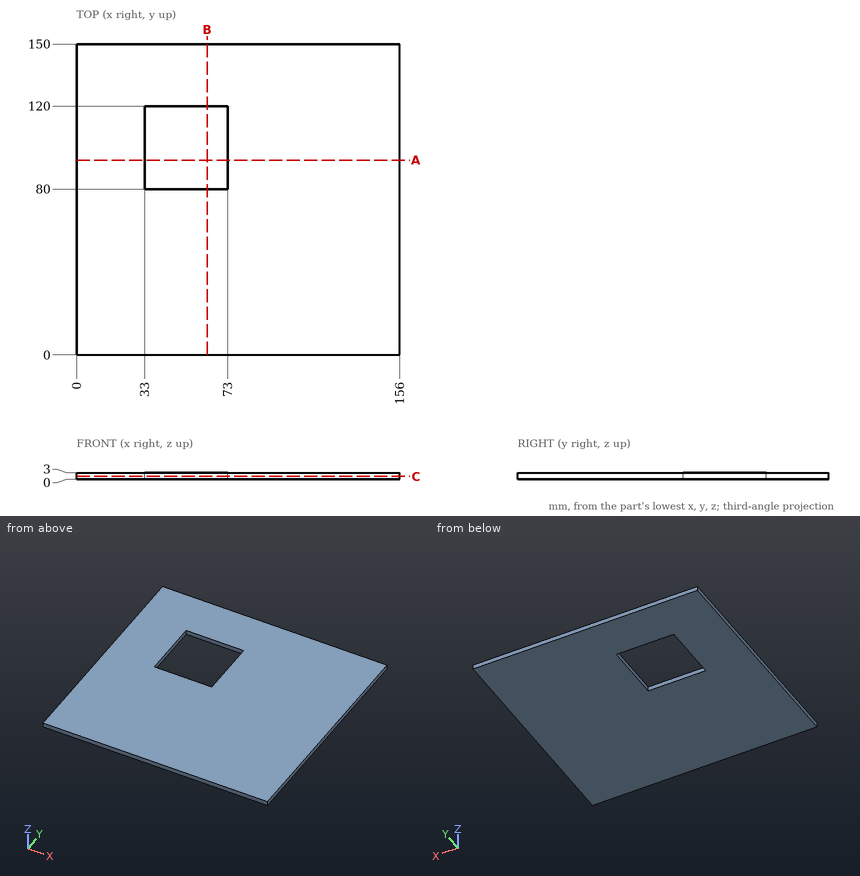
For this review, use the dimensioned drawing (mm, ordinates from the lowest corner) and the shaded views. Give positions to 0.01 mm unless a question says otherwise; leave off trailing zeros. Loops run counter-clockwise (first coordinate to the right, second up) from the corner with the lowest first, then second, coordinate; pieces in that order, holes last. Notation, with made-up numbers: (-13, -39) -> (46, -39) arc R14 cw to (46, -33) -> close; hole circle Ø10 at (40.25, -13.75). An arc over 180 degrees is marked (long way). One line per question, with ' | ' between items. Start each with the question number.
(1) We need section A-A (y = 94). State the section outline as (x, z) points.
(2) For line 1 (X direction, y = 108, z = 1.15); line 2 (Y direction, x = 60.5, z = 2.8), list the stretches that pass through material, from the lowest coordinate up.
(3) We need section C-C (z = 1.25). State the section outline as (x, y) points, and give its area (3 significant figures).
(4) We need section B-B (x = 63). State the section outline as (y, z) points.
The answers:
1) outline: (0, 0) -> (33, 0) -> (33, 3) -> (0, 3) -> close; (73, 0) -> (156, 0) -> (156, 3) -> (73, 3) -> close
2) line 1: x = 0 to 33, 73 to 156 | line 2: y = 0 to 80, 120 to 150
3) outline: (0, 0) -> (156, 0) -> (156, 150) -> (0, 150) -> close; hole (33, 80) -> (73, 80) -> (73, 120) -> (33, 120) -> close | area: 21,800 mm^2
4) outline: (0, 0) -> (80, 0) -> (80, 3) -> (0, 3) -> close; (120, 0) -> (150, 0) -> (150, 3) -> (120, 3) -> close
